Read the model definition and answer for the solid it produces. Units are mm, in the model's axes. A direction names the side the tool comes from. Round coordinates to 2 decimals unless told otherwise and drop trailing zeros. Write each loop counter-clockwise with the first axis right and the second up, starting at its lowest first coordinate (ties: lowest second). Pieces come first, ordered by that corner, then holes. Notation, with made-up numbers: (9.5, 38.25) - (38.5, 38.25) arc R23 ccw to (38.5, 57.25) - close; hole circle Ø4 at (-16.75, 37). An arc over 180 degrees is marked (long way). Answer as CSV lines item,"result". Start each with the question number.
1) Find section B-B on y = -256. Determine the outline of the cut face in (x, z).
2) Find section D-D on y = 0. Determine the outline of the cut face in (x, z), then the cut area to 3 significant figures.
3) Find section C-C on z = 177. Determine the outline of the cut face in (x, y), then the cut area to 3 significant figures.
4) Each of these flat-tipped pins is pushed along its axis until it touches: pin 1 (1.5 mm diameter, centred on y = -127, z = 324.5, fed in from +X); pin 2 (3 mm diameter, centred on y = -99.5, z = 1097, fed in from -X); pin 3 (6 mm diameter, centred on x = 10, y = 242.5, fed in from -Z). Where does it stop, or does it pass through?
5) Find section A-A on x = 0. Determine the outline of the cut face in (y, z), then the cut area to 3 significant figures.
6) For a pull along X with two mould halves and no side action, classify faces 1 (the flat face through (242.068, 168.626, -73.95)), 2 (the flat face through (-320.254, 185.303, -73.95)), 3 (the flat face through (257, 148, -150)) as +X half, -X half, draft (parallel to the pull), parting line (faces both ways), or undercut.
7) Consider line 1 along Z through (x, y) = (-76, 240); line 2 along Y through (x, z) = (-375.5, 171); line 3 along Y through (x, z) = (381, 1418). Determine where each line is inside the solid, lowest interval first.
8) Which of the six approach directions +Z, -Z, +X, -X, +Y, -Y give full straight-line access (tool end or side, diameter ignored) to faces 4 (the flat face through (190.7, 109.7, -74)), 5 (the flat face through (25, -294, -74)), 6 (the flat face through (320.604, 184.697, -73.95)), 7 (the flat face through (267.068, 125.324, -73.95))?
from build123d import *

# Parameters (mm, degrees)
F0_R            = 425
F1_DEPTH        = 1950
F2_W            = 50
F2_H            = 150
F3_DEPTH        = 150
F3_COPIES_COUNT = 3


# Not quite as in the source:
# - a pattern or mirror of a feature is missing from the dataset's text; its kind, count and spacing are read off the source's solid


with BuildPart() as f1:
    # F0 (on Top) → F1 (new body)
    with BuildSketch(Plane.XY):
        Circle(F0_R)
    extrude(amount=F1_DEPTH)

    # F2 (on face) → F3 (join)
    with BuildSketch(Plane(origin=(0, 0, 0), x_dir=(1, 0, 0), z_dir=(0, 0, -1))):
        with Locations((0, 295)):
            Rectangle(F2_W, F2_H)
    f3 = extrude(amount=F3_DEPTH)

    # F3_copies: F3 ×3 about axis
    f3_copies_axis = Axis((0, 0, 0), (0, 0, 1))
    for i in range(1, F3_COPIES_COUNT):
        add(f3.rotate(f3_copies_axis, i * 360 / F3_COPIES_COUNT))


solid = f1.part
Check values:
1,outline,"(-339.25, 0) - (-25, 0) - (-25, -150) - (25, -150) - (25, 0) - (339.25, 0) - (339.25, 1950) - (-339.25, 1950) - close"
2,outline,"(-425, 0) - (425, 0) - (425, 1950) - (-425, 1950) - close"
2,area,"1,660,000 mm^2"
3,outline,"circle Ø850 at (0, 0)"
3,area,"567,000 mm^2"
4,pin 1,"stops at x = 405.82"
4,pin 2,"stops at x = -413.55"
4,pin 3,"stops at z = 0"
5,outline,"(-425, 0) - (-370, 0) - (-370, -150) - (-220, -150) - (-220, 0) - (425, 0) - (425, 1950) - (-425, 1950) - close"
5,area,"1,680,000 mm^2"
6,face 1,"undercut"
6,face 2,"-X half"
6,face 3,"draft"
7,line 1,"z = 0 to 1950"
7,line 2,"y = -199.06 to 199.06"
7,line 3,"y = -188.32 to 188.32"
8,face 4,"-Z, -Y"
8,face 5,"-Z, +X, +Y, -Y"
8,face 6,"-Z, +X, +Y"
8,face 7,"-Z, +X, -Y"
